Input: part model. Units: mm. Frame: model coordinates. Face numbers are marked on the shaded views. A direction names the side the tool comes from. Coordinates: 2 decimals unless noted, no trailing zeros. Order: outer loops, then holes, each group sorted by start corner. A loop starts at its lowest first (then second) coordinate and runs counter-clockwise, first axis right, second up.
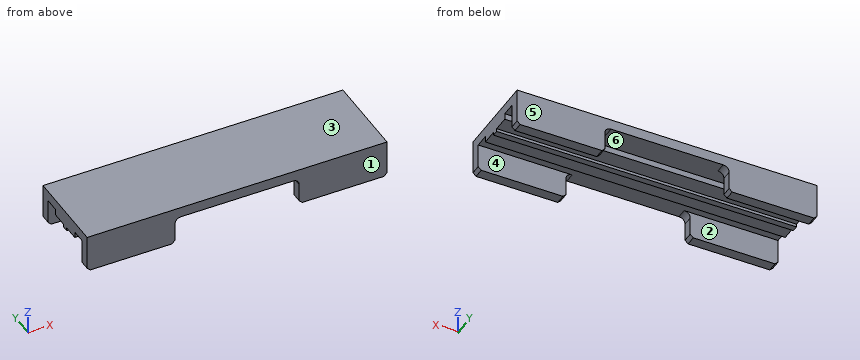
from build123d import *

# Parameters (mm, degrees)
SKETCH1_W           = 99
SKETCH1_H           = 28
BOSS_EXTRUDE1_DEPTH = 2.5
SKETCH2_W           = 29
SKETCH2_H           = 7
BOSS_EXTRUDE2_DEPTH = 3.3
FILLET1_R           = 2
SKETCH5_W           = 99
SKETCH5_H           = 9
BOSS_EXTRUDE3_DEPTH = 2
MOVE_FACE2_BY       = 2
MOVE_FACE2_2_BY     = 2
CHAMFER1_SIZE       = 1
SKETCH6_W           = 99
SKETCH6_H           = 2
BOSS_EXTRUDE4_DEPTH = 1
MOVE_FACE3_BY       = 0.9


with BuildPart() as part:
    # Sketch1 → Boss-Extrude1 (new body)
    with BuildSketch(Plane.XY):
        with Locations((75, 10)):
            Rectangle(SKETCH1_W, SKETCH1_H)
    extrude(amount=BOSS_EXTRUDE1_DEPTH)

    # Sketch2 → Boss-Extrude2 (add)
    with BuildSketch(Plane.XZ.offset(4)):
        with Locations((40, -3.5)):
            Rectangle(SKETCH2_W, SKETCH2_H)
        with Locations((110, -3.5)):
            Rectangle(SKETCH2_W, SKETCH2_H)
    extrude(amount=-BOSS_EXTRUDE2_DEPTH)

    # Fillet1
    fillet1_edges = [part.edges().sort_by_distance(p)[0] for p in [
        (54.5, -2.35, 0),
        (95.5, -2.35, 0),
    ]]
    fillet(fillet1_edges, radius=FILLET1_R)

    # Sketch5 → Boss-Extrude3 (add)
    with BuildSketch(Plane(origin=(0, 0, 0), x_dir=(-1, 0, 0), z_dir=(0, 0, -1))):
        with Locations((-75, 11.65)):
            Rectangle(SKETCH5_W, SKETCH5_H)
    extrude(amount=BOSS_EXTRUDE3_DEPTH)

    # Move Face2: a face moved outward by 2.0
    extrude(part.faces().sort_by_distance((40, -2.35, -7))[0], amount=MOVE_FACE2_BY, dir=(0, 0, -1))

    # Move Face2 2: a face moved outward by 2.0
    extrude(part.faces().sort_by_distance((110, -2.35, -7))[0], amount=MOVE_FACE2_2_BY, dir=(0, 0, -1))

    # Chamfer1
    chamfer1_edges = [part.edges().sort_by_distance(p)[0] for p in [
        (54.5, -2.35, -9),
        (25.5, -2.35, -9),
        (95.5, -2.35, -9),
        (124.5, -2.35, -9),
    ]]
    chamfer(chamfer1_edges, length=CHAMFER1_SIZE)

    # Mirror1: part across plane


with BuildPart() as part_1:
    add(part.part)
    add(part.part.mirror(Plane(origin=(0, 10, 0), x_dir=(0, 0, 1), z_dir=(0, -1, 0))))

    # Sketch6 → Boss-Extrude4 (add)
    with BuildSketch(Plane(origin=(0, 0, -2), x_dir=(-1, 0, 0), z_dir=(0, 0, -1))):
        with Locations((-75, 10)):
            Rectangle(SKETCH6_W, SKETCH6_H)
    extrude(amount=BOSS_EXTRUDE4_DEPTH)

    # Move Face3: a face moved outward by 0.9
    extrude(part_1.faces().sort_by_distance((75, 10, 2.5))[0], amount=MOVE_FACE3_BY, dir=(0, 0, 1))


solid = part_1.part
Item 1: Pin query (flat end, axial travel): pin 1 Ø6.5 at (x, y) = (61, 19) entering from -Z; pin 2 Ø1.1 at (x, z) = (59, -2.5) entering from -Y; pin 3 Ø1 at (x, z) = (90.5, -4.5) entering from +Y; pin 4 Ø1 at (x, z) = (77.5, -1) entering from +Y. Return the tip coordinate at first contact, or that it passes through.
Response values:
pin 1: stops at z = -2
pin 2: stops at y = 3.85
pin 3: passes through
pin 4: stops at y = 16.15
Item 2: Draft query along Y for the marked faces 1, 2 and 3. Return one class per face: pulls with the +Y half, pulls with the -Y half, needs draft (parallel to the pull), parting line crosses it, or undercut.
Response values:
face 1: pulls with the -Y half
face 2: undercut
face 3: needs draft
Item 3: Cut plane D-D on x = 99. Return loops of the section in (y, z).
Response values:
outline: (-4, -9) - (-0.7, -9) - (-0.7, 0) - (3.85, 0) - (3.85, -2) - (9, -2) - (9, -3) - (11, -3) - (11, -2) - (16.15, -2) - (16.15, 0) - (20.7, 0) - (20.7, -9) - (24, -9) - (24, 3.4) - (-4, 3.4) - close
Item 4: Ray query, probe 1 along Y at (x, z) = (114, -1.75); probe 2 along X at (y, z) = (-1.25, -3.5); probe 3 along Y at (x, z) = (45, -8). Return the intervals inside material, ascending.
Response values:
probe 1: y = -4 to -0.7, 3.85 to 16.15, 20.7 to 24
probe 2: x = 25.5 to 54.5, 95.5 to 124.5
probe 3: y = -4 to -0.7, 20.7 to 24
Item 5: Cut plane B-B on x = 58. Return loops of the section in (y, z).
Response values:
outline: (-4, 0) - (3.85, 0) - (3.85, -2) - (9, -2) - (9, -3) - (11, -3) - (11, -2) - (16.15, -2) - (16.15, 0) - (24, 0) - (24, 3.4) - (-4, 3.4) - close
Item 6: Cut plane C-C on y = 14.75. Return loops of the section in (x, z).
Response values:
outline: (25.5, -2) - (124.5, -2) - (124.5, 3.4) - (25.5, 3.4) - close
Item 7: Cut plane A-A on z = -6.75. Return loops of the section in (x, y).
Response values:
outline: (25.5, -4) - (54.5, -4) - (54.5, -0.7) - (25.5, -0.7) - close; (25.5, 20.7) - (54.5, 20.7) - (54.5, 24) - (25.5, 24) - close; (95.5, -4) - (124.5, -4) - (124.5, -0.7) - (95.5, -0.7) - close; (95.5, 20.7) - (124.5, 20.7) - (124.5, 24) - (95.5, 24) - close
Item 8: Access query for the marked faces 4, 5 and 6. Directions: +Z, -Z, +X, -X, +Y, -Y. A direction counts if a zero-diameter tool reaches every point of the face in a straight line with its end or side. Return the directions, or none.
Response values:
face 4: -Z, +X, -X
face 5: +Z, -Z, +X, -X, +Y
face 6: -Z
